Design review of the part built by this model. Coordinates are the model's own, in mm. Round coordinates to 2 decimals unless told otherwise and drop trailing zeros. Order: outer loops, then holes, each group sorted by start corner. A loop starts at its lowest first (then second) coordinate and runs counter-clockwise, first axis right, second up. Notation, with made-up numbers: M 25,25 L 73,25 A20 cw 73,40 Z; hole C -1.75,-15.5 d4. An arc over 180 degrees is marked long. Write each question's results on one line, items separated by ' | '. Start each with the question number.
Item 1: The part is to be moulded in two halves that separate along Y. For faces 1 (the flat face through (237.12, -23.48, 117.65)), 2 (the flat face through (221.35, -29.79, 81.85)), say which applies: +Y half, -Y half, draft (parallel to the pull), parting line (faces both ways), or undercut.
Item 2: Clearance check with flat-ended pins moving along their axes: pin 1 (8 mm diameter, centred on x = 241.5, z = 106.5, fed in from +Y); pin 2 (1 mm diameter, centred on x = 285.5, z = 93, fed in from -Y). State where each tip first meets the part, or that it passes through.
Item 3: Wall thickness on line 1 (Y direction, x = 249, z = 147.5); line 2 (Y direction, x = 190, z = 131.5): over which ranges is each line inside the solid? List them lowest first. Write a range as [from, to].
Item 4: Take a section at A-A, the plane z = 63. Write out the cut boundary in (x, y) (3 decimals).
Item 5: Take a section at B-B, the plane x = 225. Write out the cut boundary in (y, z) (3 decimals), plus the area to 3 significant figures.
```python
from build123d import *

# Parameters (mm, degrees)
BOSS_EXTRUDE1_DEPTH     = 304.8
CUT_EXTRUDE1_DEPTH      = 198.18
CUT_EXTRUDE1_DEPTH_BACK = 1
CUT_EXTRUDE2_DEPTH      = 60.305329017


with BuildPart() as part:
    # Sketch1 → Boss-Extrude1 (new body)
    with BuildSketch(Plane(origin=(0, 0, 0), x_dir=(0, 0, -1), z_dir=(1, 0, 0))):
        Polygon((0, 0), (-197.18, 0), (-162.940052328, -59.305329017), align=None)
    extrude(amount=BOSS_EXTRUDE1_DEPTH)

    # Sketch2 → Cut-Extrude1 (cut, two sides)
    with BuildSketch(Plane.XY) as cut_extrude1_sk:
        Polygon((138.684947672, -59.305329017), (301.625, 0), (0, 0), (0, -59.305329017), align=None)
        Polygon((304.8, 0), (141.859947672, -59.305329017), (304.8, -59.305329017), align=None)
    extrude(amount=CUT_EXTRUDE1_DEPTH, mode=Mode.SUBTRACT)
    extrude(cut_extrude1_sk.sketch, amount=-CUT_EXTRUDE1_DEPTH_BACK, mode=Mode.SUBTRACT)

    # Sketch3 → Cut-Extrude2 (cut, through all)
    with BuildSketch(Plane(origin=(0, 0, 0), x_dir=(1, 0, 0), z_dir=(0, 1, 0))):
        Polygon((254.596089188, -187.297424032), (301.625, -197.18), (301.625, -194.746742189), (255.085785802, -184.967070242), align=None)
        Polygon((301.625, -194.746742189), (301.625, -197.18), (304.8, -197.18), (304.8, -195.413931332), align=None)
    extrude(amount=-CUT_EXTRUDE2_DEPTH, mode=Mode.SUBTRACT)


solid = part.part
```
Results list:
1) face 1: +Y half | face 2: -Y half
2) pin 1: y = -20.43 | pin 2: y = -7.21
3) line 1: [-20.31, -19.15] | line 2: [-41.78, -40.63]
4) outline: M 238.625,-22.93 L 241.8,-22.93 L 304.8,0 L 301.625,0 Z
5) outline: M -29.045,79.8 L -27.889,76.625 L -27.889,181.078 L -29.045,180.411 Z | area: 118 mm²
